Work out the finished part from the listing and answer in its coordinate system (mm). A direction names the side the tool comes from. Round coordinates to 2 decimals unless told otherwise and drop trailing zeros. Loops run counter-clockwise (first coordinate to the right, second up) from the corner with the lowest first, then second, coordinate; pieces in that order, holes last. Notation, with made-up numbers: (34, 11.5) - (52, 11.5) arc R20 ccw to (52, 46.5) - close; hole circle Ø4 at (70.25, -23.75). An arc over 180 degrees is marked (long way). Return JSON: item names as keys, results as strings.
Autodesk Inventor part; units mm, degrees
ref_plane "YZ Plane" through (0, 0, 0) normal (1, 0, 0) x (0, 1, 0)
ref_plane "XZ Plane" through (0, 0, 0) normal (0, 1, 0) x (-1, 0, 0)
ref_plane "XY Plane" through (0, 0, 0) normal (0, 0, 1) x (1, 0, 0)
sketch "Skizze1" plane through (0, 0, 0) normal (0, 1, 0) x (-1, 0, 0)
  line L0 (0, 0) -> (30, 0)
  line L1 (30, 0) -> (30, -1000)
  line L2 (30, -1000) -> (0, -1000)
  line L3 (0, -1000) -> (0, 0)
  line L4 (0, 0) -> (-20, 0)
  line L5 (-5, -20) -> (0, -20)
  arc A0 (0, -20) -> (-20, 0) centre (-20, -20) ccw
  line L6 (30, 0) -> (30, -20)
  line L7 (30, -20) -> (35, -20)
  arc A1 (50, 0) -> (30, -20) centre (50, -20) ccw
  line L8 (50, 0) -> (50, -5)
  arc A2 (50, -5) -> (35, -20) centre (50, -20) ccw
  line L9 (0, -20) -> (-5, -20)
  arc A3 (-5, -20) -> (-20, -5) centre (-20, -20) ccw
  line L10 (35, -20) -> (35, -1000)
  line L11 (35, -1000) -> (30, -1000)
  line L12 (0, -1000) -> (-5, -1000)
  line L13 (-5, -1000) -> (-5, -20)
  line L14 (30, 0) -> (50, 0)
  line L15 (-20, -5) -> (-20, 0)
  line L16 (-20, 0) -> (0, 0)
  line L17 (0, 0) -> (0, -20)
  line L18 (0, -20) -> (-5, -20)
  line L19 (-20, -5) -> (-20, 0)
  arc A4 (0, -20) -> (-20, 0) centre (-20, -20) ccw
  line L20 (0, -20) -> (0, 0)
  line L21 (0, 0) -> (-20, 0)
  dimension "d0" = 30
  dimension "d1" = 1000
  dimension "d2" = 20
  dimension "d5" = 20
  dimension "d10" = 5
  dimension "d11" = 5
  dimension "d12" = 5
extrude "Extrusion1" add sketch "Skizze1" along normal blind 5
extrude "Extrusion2" add sketch "Skizze1" against normal blind 50 contours L3 L12 L13 L5 | L5 A3 L15 A0 | L7 L10 L11 L1 | A1 L8 A2 L7
extrude "Extrusion3" add sketch "Skizze1" against normal blind 50 contours L0 L1 L2 L3 | L3 A0 L4 | L14 A1 L1
extrude "Extrusion4" cut sketch "Skizze1" against normal blind 40 contours L0 L1 L2 L3 | L3 A0 L4 | L14 A1 L1
sketch "Skizze2" plane through (0, 0, 0) normal (0, -1, 0) x (1, 0, 0)
  arc A0 (-35, -20) -> (-50, -5) centre (-50, -20) ccw
  line L0 (5, -20) -> (5, -1000)
  line L1 (-50, -5) -> (5, -20)
  line L2 (5, -36.012) -> (-15, -36.012)
  line L3 (-35, -20) -> (-35, -1000)
  line L4 (-15, -36.012) -> (-22.5, -36.012)
  line L5 (-22.5, -36.012) -> (-7.5, -36.012)
  line L6 (-7.5, -36.012) -> (-7.5, 0)
  line L7 (-50, 0) -> (20, 0)
  line L8 (-7.5, 0) -> (-22.5, 0)
  line L9 (-22.5, 0) -> (-22.5, -1000)
  line L10 (-30, -1000) -> (0, -1000)
  line L11 (-22.5, -1000) -> (-7.5, -1000)
  line L12 (-7.5, -1000) -> (-7.5, 0)
  point P0 (0, 0)
  dimension "d21" = 20
  dimension "d22" = 15
  dimension "d23" = 15
  dimension "d24" = 15
extrude "Extrusion5" cut sketch "Skizze2" along normal blind 50 contours L9 L7 L6 L1 | L1 L6 L2 L4 L9 | L4 L2 L12 L10 L9
properties part number "Fuehrungsschiene"
1) Section B-B (z = -368) is taken. Give the vertices of the cut face in (x, y).
Verdict:
{"outline": "(-35, -50) - (-22.5, -50) - (-22.5, -40) - (-30, -40) - (-30, 0) - (0, 0) - (0, -40) - (-7.5, -40) - (-7.5, -50) - (5, -50) - (5, 5) - (-35, 5) - close"}
2) Find the intervals of material crossed by L1, parallel to X at y = -38, z = -765; L2, parallel to X at y = -43, z = -218.5; L3, parallel to Y at x = -6.5, z = -143.5, in increasing order.
Verdict:
{"L1": "x = -35 to -30, 0 to 5", "L2": "x = -35 to -22.5, -7.5 to 5", "L3": "y = -50 to -40, 0 to 5"}
3) Determine the mould class of faces 1 (the flat face through (-30, -50, -493)), 2 (the flat face through (-35, -23, -503)), 3 (the flat face through (-4, -40, -498)) for opening direction X: pulls with the +X half, pulls with the -X half, needs draft (parallel to the pull), parting line crosses it, or undercut.
Verdict:
{"face 1": "needs draft", "face 2": "pulls with the -X half", "face 3": "undercut"}
4) Flat-ended cylindrical pins translate along their axes: pin 1 (12 mm diameter, centred on y = -36.5, z = -370.5, fed in from -X); pin 2 (12 mm diameter, centred on y = -32, z = -403.5, fed in from +X); pin 3 (12 mm diameter, centred on x = -28, y = -11.5, fed in from -Z); pin 4 (1 mm diameter, centred on x = -41.5, y = -29.5, fed in from +Z). Find the tip coordinate at first contact, or state that the pin passes through.
Verdict:
{"pin 1": "stops at x = -35", "pin 2": "stops at x = 5", "pin 3": "stops at z = -1000", "pin 4": "stops at z = -1.67"}
5) Section A-A (y = -29) is taken. Give the vertices of the cut face in (x, z), and give its area (3 significant figures).
Verdict:
{"outline": "(-50, -5) arc R15 cw to (-35, -20) - (-35, -1000) - (-30, -1000) - (-30, -20) arc R20 ccw to (-50, 0) - close; (0, -1000) - (5, -1000) - (5, -20) arc R15 cw to (20, -5) - (20, 0) arc R20 ccw to (0, -20) - close", "area": "10,100 mm2"}
6) A tool of negligible diameter and unlimited length cuts with its end or side. For faces 4 (the cylindrical face through (5.703, -19.72, -6.014)), 5 (the flat face through (-30, -20, -503)), 6 (the flat face through (5, -23, -517)), from which of +Z, -Z, +X, -X, +Y, -Y can it reach the whole face along a straight path? Write none if from no direction.
Verdict:
{"face 4": "+Z", "face 5": "+Z, -Z", "face 6": "-Z, +X, +Y, -Y"}
